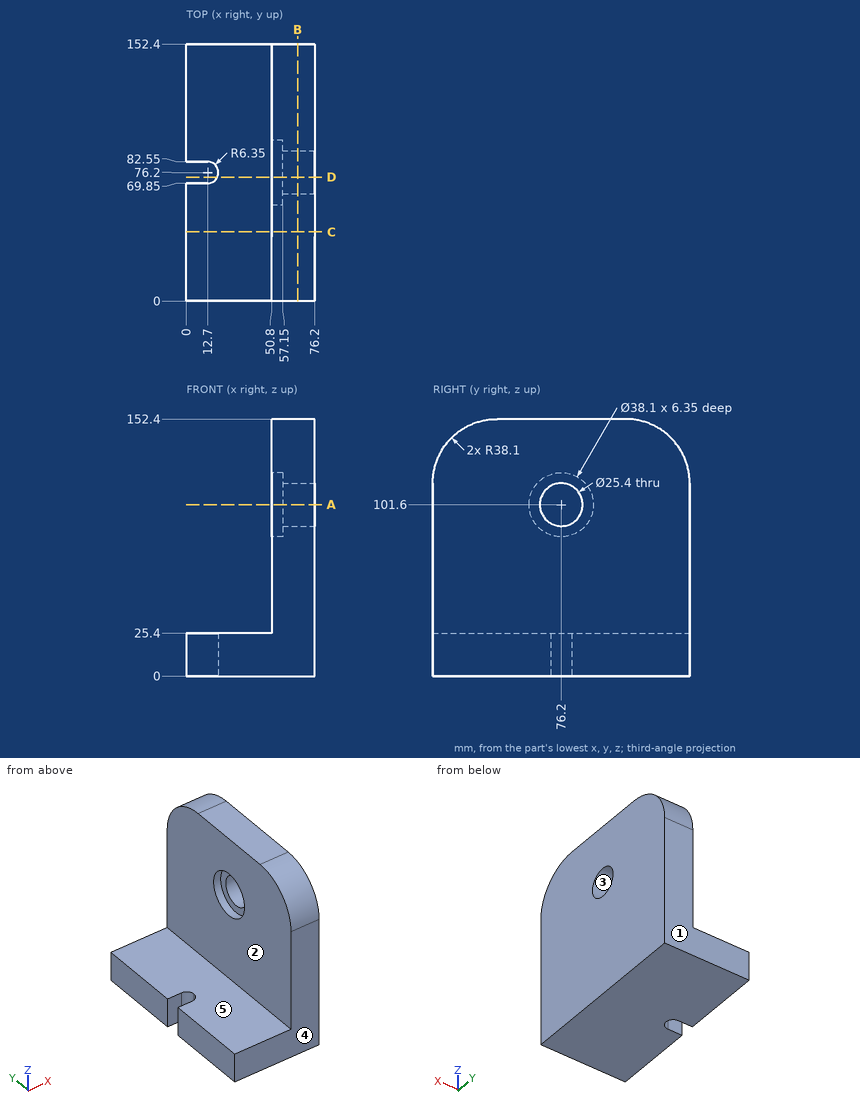
Check sheet for the drawn part. Datum: minimum x, y, z corner. Units: mm. A direction names the side the tool comes from. Give positions to 0.01 mm unless a question says otherwise; leave off trailing zeros. Order: outer loops, then holes, each group sorted by start corner. A loop starts at its lowest first (then second) coordinate and runs counter-clockwise, first axis right, second up. Notation, with made-up numbers: (25, -20.75) - (31, -20.75) arc R7 cw to (31, -7.75) - close; hole circle Ø11 at (22.25, 50.5). An arc over 180 degrees is marked (long way). Answer as a JSON object with one key per item and string values.
(1) Draft check along Y on the marked faces 3, 4 and 5. Enter one of: released by +Y, released by -Y, zero draft, split by the parting line, or undercut.
Report:
{"face 3": "undercut", "face 4": "released by -Y", "face 5": "zero draft"}
(2) Cross-section at B-B (x = 66). Record the cut outline in (y, z).
Report:
{"outline": "(0, 0) - (152.4, 0) - (152.4, 114.3) arc R38.1 ccw to (114.3, 152.4) - (38.1, 152.4) arc R38.1 ccw to (0, 114.3) - close; hole circle Ø25.4 at (76.2, 101.6)"}
(3) Depth check by flat-ended pin: pin 1 Ø1.5 at (y, z) = (112.5, 120.5) entering from -X; pin 2 Ø8 at (x, z) = (45.5, 46.5) entering from -Y. Enter the tip coordinate at first touch or a pass-through.
Report:
{"pin 1": "x = 50.8", "pin 2": "through"}
(4) Cross-section at D-D (y = 73.5). Record the cut outline in (x, z), then the cut area to 3 significant figures.
Report:
{"outline": "(18.45, 0) - (76.2, 0) - (76.2, 89.19) - (57.15, 89.19) - (57.15, 82.74) - (50.8, 82.74) - (50.8, 25.4) - (18.45, 25.4) - close; (50.8, 120.46) - (57.15, 120.46) - (57.15, 114.01) - (76.2, 114.01) - (76.2, 152.4) - (50.8, 152.4) - close", "area": "3,980 mm^2"}
(5) Tool access check on the marked faces 1 and 2. Record the directions out of +Z, -Z, +X, -X, +Y, -Y that give a thin tool (end or side, any length) a straight path to the whole face; none if there is none.
Report:
{"face 1": "+Z, -Z, +X, -X, +Y", "face 2": "+Z, -X, +Y, -Y"}
(6) Cross-section at C-C (y = 41). Record the cut outline in (x, z), then the cut area to 3 significant figures.
Report:
{"outline": "(0, 0) - (76.2, 0) - (76.2, 152.4) - (50.8, 152.4) - (50.8, 25.4) - (0, 25.4) - close", "area": "5,160 mm^2"}
(7) Cross-section at A-A (z = 101.6). Record the cut outline in (x, y), then the cut area to 3 significant figures.
Report:
{"outline": "(50.8, 0) - (76.2, 0) - (76.2, 63.5) - (57.15, 63.5) - (57.15, 57.15) - (50.8, 57.15) - close; (50.8, 95.25) - (57.15, 95.25) - (57.15, 88.9) - (76.2, 88.9) - (76.2, 152.4) - (50.8, 152.4) - close", "area": "3,150 mm^2"}
(8) Material ranges on line 1 (Z direction, x = 71.5, y = 76.2); line 2 (Y direction, x = 54, z = 101); line 3 (Z direction, x = 54.75, y = 76.2), recorded low to high.
Report:
{"line 1": "0 to 88.9, 114.3 to 152.4", "line 2": "0 to 57.16, 95.24 to 152.4", "line 3": "0 to 82.55, 120.65 to 152.4"}
